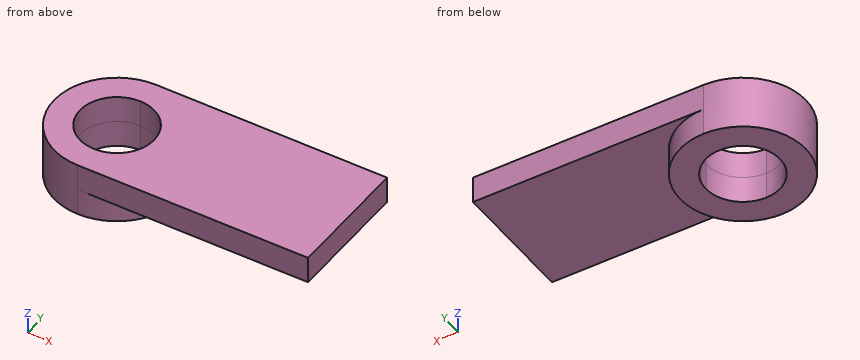
from build123d import *

# Parameters (mm, degrees)
F1_DEPTH = 6.35
F2_DEPTH = 6.35


with BuildPart() as f1:
    # F0 (on Top) → F1 (new body)
    with BuildSketch(Plane.XY):
        with BuildLine():
            ThreePointArc((-12.4036967908, 0), (-16.7460770157, 10.483433232), (-27.2295102477, 14.8258134569))
            Line((-27.2295102477, 14.8258134569), (-27.2295102477, 8.7676478071))
            ThreePointArc((-27.2295102477, 8.7676478071), (-21.0298470283, 6.1996632194), (-18.4618624406, 0))
            ThreePointArc((-18.4618624406, 0), (-21.0298470283, -6.1996632194), (-27.2295102477, -8.7676478071))
            Line((-27.2295102477, -8.7676478071), (-27.2295102477, -14.8258134569))
            ThreePointArc((-27.2295102477, -14.8258134569), (-16.7460770157, -10.483433232), (-12.4036967908, 0))
        make_face()
        with BuildLine():
            Line((27.2295102477, 14.8258134569), (-27.2295102477, 14.8258134569))
            ThreePointArc((-27.2295102477, 14.8258134569), (-16.7460770157, 10.483433232), (-12.4036967908, 0))
            ThreePointArc((-12.4036967908, 0), (-16.7460770157, -10.483433232), (-27.2295102477, -14.8258134569))
            Line((-27.2295102477, -14.8258134569), (27.2295102477, -14.8258134569))
            Line((27.2295102477, -14.8258134569), (27.2295102477, 14.8258134569))
        make_face()
        with BuildLine():
            Line((-27.2295102477, 8.7676478071), (-27.2295102477, 14.8258134569))
            ThreePointArc((-27.2295102477, 14.8258134569), (-42.0553237046, 0), (-27.2295102477, -14.8258134569))
            Line((-27.2295102477, -14.8258134569), (-27.2295102477, -8.7676478071))
            ThreePointArc((-27.2295102477, -8.7676478071), (-35.9971580548, 0), (-27.2295102477, 8.7676478071))
        make_face()
    extrude(amount=F1_DEPTH)

    # F0 (on Top) → F2 (join)
    with BuildSketch(Plane.XY):
        with BuildLine():
            Line((-27.2295102477, 8.7676478071), (-27.2295102477, 14.8258134569))
            ThreePointArc((-27.2295102477, 14.8258134569), (-42.0553237046, 0), (-27.2295102477, -14.8258134569))
            Line((-27.2295102477, -14.8258134569), (-27.2295102477, -8.7676478071))
            ThreePointArc((-27.2295102477, -8.7676478071), (-35.9971580548, 0), (-27.2295102477, 8.7676478071))
        make_face()
        with BuildLine():
            ThreePointArc((-12.4036967908, 0), (-16.7460770157, 10.483433232), (-27.2295102477, 14.8258134569))
            Line((-27.2295102477, 14.8258134569), (-27.2295102477, 8.7676478071))
            ThreePointArc((-27.2295102477, 8.7676478071), (-21.0298470283, 6.1996632194), (-18.4618624406, 0))
            ThreePointArc((-18.4618624406, 0), (-21.0298470283, -6.1996632194), (-27.2295102477, -8.7676478071))
            Line((-27.2295102477, -8.7676478071), (-27.2295102477, -14.8258134569))
            ThreePointArc((-27.2295102477, -14.8258134569), (-16.7460770157, -10.483433232), (-12.4036967908, 0))
        make_face()
    extrude(amount=-F2_DEPTH)


solid = f1.part
Input: part model. Units: mm. Frame: model coordinates. Give positions to 0.01 mm unless a question says otherwise; leave off trailing zeros. Write each loop counter-clockwise with the first axis right and the second up, starting at its lowest first coordinate (ties: lowest second). Pieces come first, ordered by that corner, then holes. Notation, with made-up numbers: M -8,3.5 L 12,3.5 A26 cw 12,36.5 Z; hole C 67.25,71 d2. An arc over 180 degrees is marked long. Use one line per item in the form item = value.
1. First-contact query: P1, Ø1, axis at x = 13, z = -1, coming from the -Y side; P2, Ø15, axis at x = -6.5, y = 1.5, coming from the -Z side; P3, Ø3, axis at x = 2.5, y = -0.5, coming from the -Z side; P4, Ø1, axis at y = 8.5, z = -1, coming from the +X side. Flat tips, straight axial feed; report the tip coordinate or a pass-through.
Outcome:
P1 = through
P2 = -6.35
P3 = 0
P4 = -14.75
2. Cut plane D-D on x = -4. Return loops of the section in (y, z), and give its area (3 significant figures).
Outcome:
outline = M -14.83,0 L 14.83,0 L 14.83,6.35 L -14.83,6.35 Z
area = 188 mm²
3. Cut plane A-A on z = -3. Return loops of the section in (x, y), and give its area (3 significant figures).
Outcome:
outline = C -27.23,0 d29.65; hole C -27.23,0 d17.54
area = 449 mm²
4. Ray query, L1, parallel to X at y = -4, z = -2.5; L2, parallel to Z at x = 2, y = 13.5; L3, parallel to X at y = -0.25, z = -2.5. Return the intervals inside material, ascending.
Outcome:
L1 = -41.51 to -35.03, -19.43 to -12.95
L2 = 0 to 6.35
L3 = -42.05 to -35.99, -18.47 to -12.41
5. Cut plane C-C on x = -19.5. Return loops of the section in (y, z).
Outcome:
outline = M -14.83,0 L -12.65,0 L -12.65,-6.35 L -4.14,-6.35 L -4.14,6.35 L -14.83,6.35 Z; M 4.14,-6.35 L 12.65,-6.35 L 12.65,0 L 14.83,0 L 14.83,6.35 L 4.14,6.35 Z
6. Cut plane B-B on y = -5.25. Return loops of the section in (x, z).
Outcome:
outline = M -41.09,-6.35 L -34.25,-6.35 L -34.25,6.35 L -41.09,6.35 Z; M -20.21,-6.35 L -13.36,-6.35 L -13.36,0 L 27.23,0 L 27.23,6.35 L -20.21,6.35 Z
